Geometry: final body of the model. Coordinates: model frame, mm. A direction names the side the tool comes from. Coordinates: 2 decimals unless noted, no trailing zeros. Order: outer loops, then holes, each group sorted by start corner. A loop starts at its lowest first (then second) coordinate and runs counter-clockwise, first axis right, second up. Notation, with made-up numbers: M -40,54.25 L 19,54.25 A28 cw 19,86.25 Z; hole C 27,-14 d9. An arc over 180 degrees is marked long. Use CSV: the item, a comma, the result in double quotes. Start each with the question number.
1. Section query A-A on z = 0. Return the cut outline in (x, y).
2. Material intervals for line 1 (X direction, y = 33, z = 0); line 2 (Z direction, x = 7, y = 44); line 3 (X direction, y = 14, z = 4.5), sorted ascending.
3. First-contact query: P1, Ø1.5, axis at x = -2, y = 11, coming from the -Z side; P2, Ø0.5, axis at x = -9, y = 29, coming from the +Z side; P3, Ø4, axis at y = 13.5, z = 1.5, coming from the -X side; P4, Ø4, axis at x = 0, z = 0, coming from the +Y side. Flat tips, straight axial feed; report the tip coordinate or a pass-through.
4. Pull-direction query (Z, two-part tool) for faces 4 (the flat face through (-5.21, 24.65, -4.15)), 5 (the cylindrical face through (9.43, 24.65, 9.4)), 6 (the flat face through (10, 25, 6)); classes: pulls with the +Z half, pulls with the -Z half, needs draft (parallel to the pull), parting line crosses it, or undercut.
5. Set-up query: faces 1 (the flat face through (5.25, 24.65, -4.19)), 2 (the cylindrical face through (-9.4, 24.65, 9.43)), 3 (the flat face through (0, 25, 3.9)). Return all of +Z, -Z, +X, -X, +Y, -Y with unobstructed straight access to the full face (end or side cutting, diameter ignored); none if empty.
6. Section query B-B on x = 0. Return the cut outline in (y, z).
from build123d import *

# Parameters (mm, degrees)
SKETCH_1_R      = 2.5
EXTRUDE_1_DEPTH = 50


with BuildPart() as part:
    # 草图1 → 凸台-拉伸1 (new body)
    with BuildSketch(Plane(origin=(0, 0, 0), x_dir=(1, 0, 0), z_dir=(0, 1, 0))):
        with BuildLine():
            Line((3.1, 8.8), (3.1, 9.4))
            ThreePointArc((3.1, 9.4), (3.275735931, 9.824264069), (3.7, 10))
            Line((3.7, 10), (8, 10))
            ThreePointArc((8, 10), (9.414213562, 9.414213562), (10, 8))
            Line((10, 8), (10, 3.7))
            ThreePointArc((10, 3.7), (9.824264069, 3.275735931), (9.4, 3.1))
            Line((9.4, 3.1), (8.8, 3.1))
            ThreePointArc((8.8, 3.1), (8.375735931, 3.275735931), (8.2, 3.7))
            Line((8.2, 3.7), (8.2, 4.9))
            ThreePointArc((8.2, 4.9), (8.024264069, 5.324264069), (7.6, 5.5))
            Line((7.6, 5.5), (6.809188309, 5.5))
            ThreePointArc((6.809188309, 5.5), (6.57957825, 5.45432772), (6.38492424, 5.324264069))
            Line((6.38492424, 5.324264069), (4.075735931, 3.01507576))
            ThreePointArc((4.075735931, 3.01507576), (3.94567228, 2.82042175), (3.9, 2.590811691))
            Line((3.9, 2.590811691), (3.9, 0))
            Line((3.9, 0), (3.9, -2.590811691))
            ThreePointArc((3.9, -2.590811691), (3.94567228, -2.82042175), (4.075735931, -3.01507576))
            Line((4.075735931, -3.01507576), (6.38492424, -5.324264069))
            ThreePointArc((6.38492424, -5.324264069), (6.57957825, -5.45432772), (6.809188309, -5.5))
            Line((6.809188309, -5.5), (7.6, -5.5))
            ThreePointArc((7.6, -5.5), (8.024264069, -5.324264069), (8.2, -4.9))
            Line((8.2, -4.9), (8.2, -3.7))
            ThreePointArc((8.2, -3.7), (8.375735931, -3.275735931), (8.8, -3.1))
            Line((8.8, -3.1), (9.4, -3.1))
            ThreePointArc((9.4, -3.1), (9.824264069, -3.275735931), (10, -3.7))
            Line((10, -3.7), (10, -8))
            ThreePointArc((10, -8), (9.414213562, -9.414213562), (8, -10))
            Line((8, -10), (3.7, -10))
            ThreePointArc((3.7, -10), (3.275735931, -9.824264069), (3.1, -9.4))
            Line((3.1, -9.4), (3.1, -8.8))
            ThreePointArc((3.1, -8.8), (3.275735931, -8.375735931), (3.7, -8.2))
            Line((3.7, -8.2), (4.9, -8.2))
            ThreePointArc((4.9, -8.2), (5.324264069, -8.024264069), (5.5, -7.6))
            Line((5.5, -7.6), (5.5, -6.809188309))
            ThreePointArc((5.5, -6.809188309), (5.45432772, -6.57957825), (5.324264069, -6.38492424))
            Line((5.324264069, -6.38492424), (3.01507576, -4.075735931))
            ThreePointArc((3.01507576, -4.075735931), (2.82042175, -3.94567228), (2.590811691, -3.9))
            Line((2.590811691, -3.9), (0, -3.9))
            Line((0, -3.9), (-2.590811691, -3.9))
            ThreePointArc((-2.590811691, -3.9), (-2.82042175, -3.94567228), (-3.01507576, -4.075735931))
            Line((-3.01507576, -4.075735931), (-5.324264069, -6.38492424))
            ThreePointArc((-5.324264069, -6.38492424), (-5.45432772, -6.57957825), (-5.5, -6.809188309))
            Line((-5.5, -6.809188309), (-5.5, -7.6))
            ThreePointArc((-5.5, -7.6), (-5.324264069, -8.024264069), (-4.9, -8.2))
            Line((-4.9, -8.2), (-3.7, -8.2))
            ThreePointArc((-3.7, -8.2), (-3.275735931, -8.375735931), (-3.1, -8.8))
            Line((-3.1, -8.8), (-3.1, -9.4))
            ThreePointArc((-3.1, -9.4), (-3.275735931, -9.824264069), (-3.7, -10))
            Line((-3.7, -10), (-8, -10))
            ThreePointArc((-8, -10), (-9.414213562, -9.414213562), (-10, -8))
            Line((-10, -8), (-10, -3.7))
            ThreePointArc((-10, -3.7), (-9.824264069, -3.275735931), (-9.4, -3.1))
            Line((-9.4, -3.1), (-8.8, -3.1))
            ThreePointArc((-8.8, -3.1), (-8.375735931, -3.275735931), (-8.2, -3.7))
            Line((-8.2, -3.7), (-8.2, -4.9))
            ThreePointArc((-8.2, -4.9), (-8.024264069, -5.324264069), (-7.6, -5.5))
            Line((-7.6, -5.5), (-6.809188309, -5.5))
            ThreePointArc((-6.809188309, -5.5), (-6.57957825, -5.45432772), (-6.38492424, -5.324264069))
            Line((-6.38492424, -5.324264069), (-4.075735931, -3.01507576))
            ThreePointArc((-4.075735931, -3.01507576), (-3.94567228, -2.82042175), (-3.9, -2.590811691))
            Line((-3.9, -2.590811691), (-3.9, 0))
            Line((-3.9, 0), (-3.9, 2.590811691))
            ThreePointArc((-3.9, 2.590811691), (-3.94567228, 2.82042175), (-4.075735931, 3.01507576))
            Line((-4.075735931, 3.01507576), (-6.38492424, 5.324264069))
            ThreePointArc((-6.38492424, 5.324264069), (-6.57957825, 5.45432772), (-6.809188309, 5.5))
            Line((-6.809188309, 5.5), (-7.6, 5.5))
            ThreePointArc((-7.6, 5.5), (-8.024264069, 5.324264069), (-8.2, 4.9))
            Line((-8.2, 4.9), (-8.2, 3.7))
            ThreePointArc((-8.2, 3.7), (-8.375735931, 3.275735931), (-8.8, 3.1))
            Line((-8.8, 3.1), (-9.4, 3.1))
            ThreePointArc((-9.4, 3.1), (-9.824264069, 3.275735931), (-10, 3.7))
            Line((-10, 3.7), (-10, 8))
            ThreePointArc((-10, 8), (-9.414213562, 9.414213562), (-8, 10))
            Line((-8, 10), (-3.7, 10))
            ThreePointArc((-3.7, 10), (-3.275735931, 9.824264069), (-3.1, 9.4))
            Line((-3.1, 9.4), (-3.1, 8.8))
            ThreePointArc((-3.1, 8.8), (-3.275735931, 8.375735931), (-3.7, 8.2))
            Line((-3.7, 8.2), (-4.9, 8.2))
            ThreePointArc((-4.9, 8.2), (-5.324264069, 8.024264069), (-5.5, 7.6))
            Line((-5.5, 7.6), (-5.5, 6.809188309))
            ThreePointArc((-5.5, 6.809188309), (-5.45432772, 6.57957825), (-5.324264069, 6.38492424))
            Line((-5.324264069, 6.38492424), (-3.01507576, 4.075735931))
            ThreePointArc((-3.01507576, 4.075735931), (-2.82042175, 3.94567228), (-2.590811691, 3.9))
            Line((-2.590811691, 3.9), (0, 3.9))
            Line((0, 3.9), (2.590811691, 3.9))
            ThreePointArc((2.590811691, 3.9), (2.82042175, 3.94567228), (3.01507576, 4.075735931))
            Line((3.01507576, 4.075735931), (5.324264069, 6.38492424))
            ThreePointArc((5.324264069, 6.38492424), (5.45432772, 6.57957825), (5.5, 6.809188309))
            Line((5.5, 6.809188309), (5.5, 7.6))
            ThreePointArc((5.5, 7.6), (5.324264069, 8.024264069), (4.9, 8.2))
            Line((4.9, 8.2), (3.7, 8.2))
            ThreePointArc((3.7, 8.2), (3.275735931, 8.375735931), (3.1, 8.8))
        make_face()
        with Locations(Location((0, 0, 0), (0, 0, 270))):
            Circle(SKETCH_1_R, mode=Mode.SUBTRACT)
    extrude(amount=EXTRUDE_1_DEPTH)


solid = part.part
Results list:
1,outline,"M -3.9,0 L -2.5,0 L -2.5,50 L -3.9,50 Z; M 2.5,0 L 3.9,0 L 3.9,50 L 2.5,50 Z"
2,line 1,"x = -3.9 to -2.5, 2.5 to 3.9"
2,line 2,"z = -10 to -5.5, 5.5 to 10"
2,line 3,"x = -10 to -8.2, -5.56 to -3.44, 3.44 to 5.56, 8.2 to 10"
3,P1,"stops at z = -3.92"
3,P2,"stops at z = 9.85"
3,P3,"stops at x = -9.97"
3,P4,"passes through"
4,face 4,"undercut"
4,face 5,"pulls with the +Z half"
4,face 6,"needs draft"
5,face 1,"+Y, -Y"
5,face 2,"+Z, -X, +Y, -Y"
5,face 3,"+Z, +Y, -Y"
6,outline,"M 0,-3.9 L 50,-3.9 L 50,-2.5 L 0,-2.5 Z; M 0,2.5 L 50,2.5 L 50,3.9 L 0,3.9 Z"
